Part model, mm, in its own coordinate system. Round coordinates to 2 decimals unless told otherwise and drop trailing zeros. Loops run counter-clockwise (first coordinate to the right, second up) from the corner with the lowest first, then second, coordinate; pieces in that order, holes last. Notation, with made-up numbers: (57, 86.5) - (69, 86.5) arc R19 cw to (69, 116.5) - close; hole circle Ø6 at (36, 8). An arc over 180 degrees is marked (long way). Put each result on its own line as item: value.
Autodesk Inventor part; units mm, degrees
ref_plane "YZ Plane" through (0, 0, 0) normal (1, 0, 0) x (0, 1, 0)
ref_plane "XZ Plane" through (0, 0, 0) normal (0, 1, 0) x (-1, 0, 0)
ref_plane "XY Plane" through (0, 0, 0) normal (0, 0, 1) x (1, 0, 0)
sketch "Sketch1" plane through (0, 0, 0) normal (0, 1, 0) x (-1, 0, 0)
  line L0 (0, 0) -> (0, -95)
  line L1 (0, -95) -> (-95, -95)
  line L2 (-95, -95) -> (-95, -70) construction
  line L3 (-95, -70) -> (-25, -70)
  line L4 (-25, -70) -> (-25, 0)
  line L5 (-25, 0) -> (0, 0)
  circle A0 centre (-12.5, -20) radius 2.75
  line L6 (-12.5, 0) -> (-12.5, -95) construction
  circle A1 centre (-12.5, -40) radius 2.75
  circle A2 centre (-12.5, -60) radius 2.75
  line L7 (-95, -82.5) -> (0, -82.5) construction
  circle A3 centre (-35, -82.5) radius 2.75
  circle A4 centre (-55, -82.5) radius 2.75
  circle A5 centre (-75, -82.5) radius 2.75
  circle A6 centre (-12.5, -30) radius 2.75
  circle A7 centre (-12.5, -50) radius 2.75
  circle A8 centre (-12.5, -70) radius 2.75
  line L8 (-400, -139.4226) -> (-400, 36.9661) construction
  line L9 (-800, 0) -> (-800, -95)
  line L10 (-800, -95) -> (-705, -95)
  line L11 (-705, -95) -> (-705, -70) construction
  line L12 (-705, -70) -> (-775, -70)
  line L13 (-775, -70) -> (-775, 0)
  line L14 (-775, 0) -> (-800, 0)
  circle A9 centre (-787.5, -20) radius 2.75
  line L15 (-787.5, 0) -> (-787.5, -95) construction
  circle A10 centre (-787.5, -40) radius 2.75
  circle A11 centre (-787.5, -60) radius 2.75
  line L16 (-705, -82.5) -> (-800, -82.5) construction
  circle A12 centre (-765, -82.5) radius 2.75
  circle A13 centre (-745, -82.5) radius 2.75
  circle A14 centre (-725, -82.5) radius 2.75
  circle A15 centre (-787.5, -30) radius 2.75
  circle A16 centre (-787.5, -50) radius 2.75
  circle A17 centre (-787.5, -70) radius 2.75
  line L17 (-95, -95) -> (-705, -95)
  line L18 (-705, -70) -> (-95, -70)
  dimension "d0" = 25
  dimension "d1" = 70
  dimension "d2" = 25
  dimension "d3" = 70
  dimension "d4" = 5.5
  dimension "d5" = 20
  dimension "d6" = 5.5
  dimension "d7" = 5.5
  dimension "d8" = 20
  dimension "d9" = 20
  dimension "d12" = 5.5
  dimension "d13" = 35
  dimension "d14" = 5.5
  dimension "d15" = 20
  dimension "d16" = 5.5
  dimension "d17" = 20
  dimension "d22" = 10
  dimension "d28" = 400
extrude "Extrusion1" add sketch "Sketch1" along normal blind 4
fillet "Fillet1" radius 20 2 edges at (25, 2, -70) (775, 2, -70)
properties part number "Brace 1" material "CFRP"
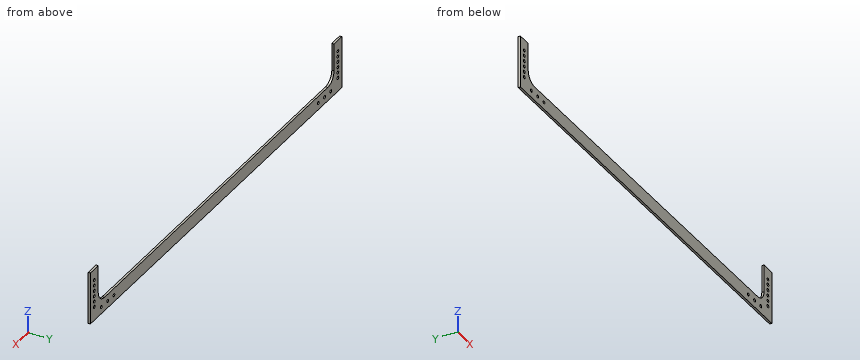
1. Band-saw the part on B-B (x = 194). List the corners of the cut face in (y, z).
A:
outline: (0, -95) - (4, -95) - (4, -70) - (0, -70) - close
2. Probe line 1 along X through (y, z) = (2.35, -29.5); line 2 along Z through (x, y) = (765, 3); line 3 along X through (y, z) = (3.5, -6). List the from-to ranges inside material, lowest first. Write a range as [from, to].
A:
line 1: x = [0, 9.8], [15.2, 25], [775, 784.8], [790.2, 800]
line 2: z = [-95, -85.25], [-79.75, -67.32]
line 3: x = [0, 25], [775, 800]
3. Band-saw the part on A-A (y = 0.7). Give the number of separate pieces and of enclosed holes in the cut face, plus the area to 3 significant figures.
A:
separate pieces: 1
enclosed holes: 18
area: 23,200 mm²
